```python
from build123d import *

# Parameters (mm, degrees)
BOSS_EXTRUDE1_DEPTH = 2
SKETCH2_W           = 3
SKETCH2_H           = 58
BOSS_EXTRUDE2_DEPTH = 3
SKETCH3_W           = 12
SKETCH3_H           = 15.5
SKETCH3_W_2         = 30
SKETCH3_H_2         = 58
BOSS_EXTRUDE3_DEPTH = 2


with BuildPart() as part:
    # Sketch1 → Boss-Extrude1 (new body)
    with BuildSketch(Plane(origin=(0, 0, 0), x_dir=(1, 0, 0), z_dir=(0, 1, 0))):
        Polygon((-22.5, 30), (42.5, 30), (42.5, -30), (-22.5, -30), (-22.5, -45), (-42.5, -45), (-42.5, -30), (-42.5, 30), (-42.5, 45), (-22.5, 45), align=None)
    extrude(amount=BOSS_EXTRUDE1_DEPTH)

    # Sketch2 → Boss-Extrude2 (add)
    with BuildSketch(Plane.XZ):
        Polygon((-42.5, -45), (-39.5, -45), (-39.5, -32.5), (-30.5, -32.5), (-30.5, -29.5), (-40.524301108, -29.5), (-42.5, -29.5), align=None)
        with Locations((-22.5, 0)):
            Rectangle(SKETCH2_W, SKETCH2_H)
        Polygon((-42.5, 45), (-39.5, 45), (-39.5, 32.5), (-30.5, 32.5), (-30.5, 29.5), (-40.524301108, 29.5), (-42.5, 29.5), align=None)
    extrude(amount=BOSS_EXTRUDE2_DEPTH)

    # Sketch3 → Boss-Extrude3 (add)
    with BuildSketch(Plane.XZ.offset(3)):
        with Locations((-36.5, 37.25)):
            Rectangle(SKETCH3_W, SKETCH3_H)
        with Locations((-36.5, -37.25)):
            Rectangle(SKETCH3_W, SKETCH3_H)
        with Locations((-9, 0)):
            Rectangle(SKETCH3_W_2, SKETCH3_H_2)
    extrude(amount=BOSS_EXTRUDE3_DEPTH)


solid = part.part
```
The model under review builds one solid part; all positions refer to its coordinate system, in mm. A direction names the side the tool comes from. Round coordinates to 2 decimals unless told otherwise and drop trailing zeros. Order: outer loops, then holes, each group sorted by start corner. A loop starts at its lowest first (then second) coordinate and runs counter-clockwise, first axis right, second up.
(1) Wall thickness on L1, parallel to Y at x = -33, z = -33; L2, parallel to Z at x = -32, y = -4; L3, parallel to Z at x = 13.5, y = 0.75: over which ranges is each line inside the solid? List them lowest first.
Working result:
L1: y = -5 to -3, 0 to 2
L2: z = -45 to -29.5, 29.5 to 45
L3: z = -30 to 30
(2) Take a section at B-B, the plane x = 4. State the section outline as (y, z) points, plus the area to 3 significant figures.
Working result:
outline: (-5, -29) - (-3, -29) - (-3, 29) - (-5, 29) - close; (0, -30) - (2, -30) - (2, 30) - (0, 30) - close
area: 236 mm2
(3) Take a section at C-C, the plane x = -33. State the section outline as (y, z) points, plus the area to 3 significant figures.
Working result:
outline: (-5, -45) - (-3, -45) - (-3, -32.5) - (0, -32.5) - (0, -45) - (2, -45) - (2, 45) - (0, 45) - (0, 32.5) - (-3, 32.5) - (-3, 45) - (-5, 45) - (-5, 29.5) - (0, 29.5) - (0, -29.5) - (-5, -29.5) - close
area: 260 mm2
(4) Tool access review of faces 1 (the face through (-35, -1, -32.5)), 2 (the face through (-24, -2, 0)), 3 (the face through (-35, -1, 32.5)): name each direction out of +Z, -Z, +X, -X, +Y, -Y from which nothing blocks a thin tool from reaching the whole face with its end or side.
Working result:
face 1: -Z, +X
face 2: +Z, -Z, -X, -Y
face 3: +Z, +X
(5) Take a section at D-D, the plane z = -8. State the section outline as (x, y) points.
Working result:
outline: (-42.5, 0) - (-24, 0) - (-24, -5) - (6, -5) - (6, -3) - (-21, -3) - (-21, 0) - (42.5, 0) - (42.5, 2) - (-42.5, 2) - close
(6) For P1, Ø1, axis at x = -26, y = -3, coming from the -Z side; P2, Ø2.5, axis at y = -1, z = -41, coming from the +X side; P3, Ø4, axis at y = -3.5, z = -2, coming from the -X side; P4, Ø1.5, axis at y = -2, z = -2, coming from the +X side, all flat-tipped, find the tip position at first contact; note any pin that passes through.
Working result:
P1: passes through
P2: stops at x = -22.5
P3: stops at x = -24
P4: stops at x = -21
(7) Take a section at A-A, the plane y = -1. State the section outline as (x, z) points.
Working result:
outline: (-42.5, -45) - (-39.5, -45) - (-39.5, -32.5) - (-30.5, -32.5) - (-30.5, -29.5) - (-42.5, -29.5) - close; (-42.5, 29.5) - (-30.5, 29.5) - (-30.5, 32.5) - (-39.5, 32.5) - (-39.5, 45) - (-42.5, 45) - close; (-24, -29) - (-21, -29) - (-21, 29) - (-24, 29) - close
